The model under review builds one solid part; all positions refer to its coordinate system, in mm. Coordinates: 2 decimals unless noted, no trailing zeros. Loops run counter-clockwise (first coordinate to the right, second up) from the corner with the lowest first, then second, coordinate; pieces in that order, holes last. Notation, with made-up numbers: M 66,24 L 77,24 A13 ccw 77,28 Z; hole C 81.5,-20 d6. An arc over 180 degrees is marked long. Write item = value, one per line. Start each with the question number.
Q1. We need section A-A on x = 82.5. Give the boundary of the cut face in (y, z), and give its area (3 significant figures).
Q2. We need section B-B on z = 0.95. Count the separate pieces of the cut face and the enclosed holes in it, and give its area (3 significant figures).
Q3. Wall thickness on probe 1 along Y at (x, z) = (-24.5, 0.85); probe 2 along Y at (x, z) = (-123.5, 0.55) (3 decimals); probe 3 along Y at (x, z) = (-7.5, 0.65): over which ranges is each line inside the solid? List them lowest first.
Q4. Clearance check with a flat-ended pin moving along its axis: pin 1 Ø1 at (y, z) = (43, 1) entering from -X. State where the tip first meets the part, or that it passes through.
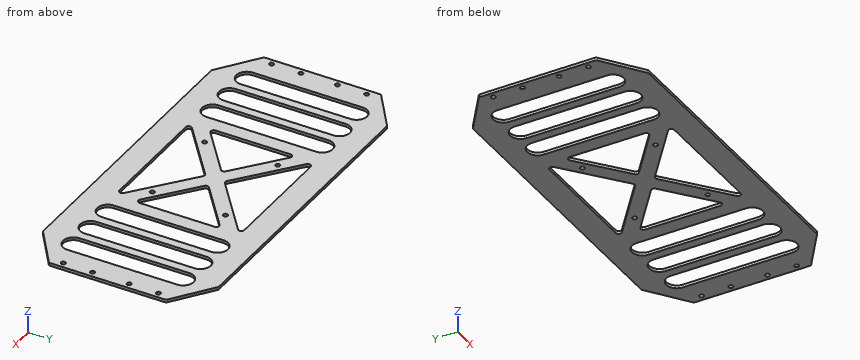
from build123d import *

# Parameters (mm, degrees)
EXTRUDE_1_DEPTH          = 2
SKETCH_2_R               = 1.525
CUT_EXTRUDE_1_DEPTH      = 1
CUT_EXTRUDE_1_DEPTH_BACK = 3
CUT_EXTRUDE_START        = -3
SKETCH_3_R               = 1.525
CUT_EXTRUDE_2_DEPTH      = 4
CUT_EXTRUDE_3_DEPTH      = 1
CUT_EXTRUDE_3_DEPTH_BACK = 3
FILLET_1_R               = 2
CUT_EXTRUDE_4_DEPTH      = 4
FILLET_2_R               = 2


with BuildPart() as part:
    # 草图1 → 凸台-拉伸1 (new body)
    with BuildSketch(Plane.XY):
        Polygon((-100, 60), (-127.5, 40), (-127.5, -40), (-100, -60), (100, -60), (127.5, -40), (127.5, 40), (100, 60), align=None)
    extrude(amount=EXTRUDE_1_DEPTH)

    # 草图2 → 切除-拉伸1 (cut, two sides)
    with BuildSketch(Plane(origin=(0, 0, 0), x_dir=(-1, 0, 0), z_dir=(0, 0, -1))) as cut_extrude_1_sk:
        with Locations((31, -25)):
            Circle(SKETCH_2_R)
        with Locations((-31, -25)):
            Circle(SKETCH_2_R)
        with Locations((-31, 25)):
            Circle(SKETCH_2_R)
        with Locations((31, 25)):
            Circle(SKETCH_2_R)
    extrude(amount=CUT_EXTRUDE_1_DEPTH, mode=Mode.SUBTRACT)
    extrude(cut_extrude_1_sk.sketch, amount=-CUT_EXTRUDE_1_DEPTH_BACK, mode=Mode.SUBTRACT)

    # 草图3 → 切除-拉伸2 (cut)
    with BuildSketch(Plane.XY.offset(2).offset(CUT_EXTRUDE_START)):
        with Locations((-123.5, -32.5)):
            Circle(SKETCH_3_R)
        with Locations((-123.5, -12.5)):
            Circle(SKETCH_3_R)
        with Locations((-123.5, 12.5)):
            Circle(SKETCH_3_R)
        with Locations((-123.5, 32.5)):
            Circle(SKETCH_3_R)
    cut_extrude_2 = extrude(amount=CUT_EXTRUDE_2_DEPTH, mode=Mode.SUBTRACT)

    # 镜向1: 切除-拉伸2 across plane
    add(cut_extrude_2.mirror(Plane(origin=(0, 0, 0), x_dir=(0, 0, 1), z_dir=(1, 0, 0))), mode=Mode.SUBTRACT)

    # 草图4 → 切除-拉伸3 (cut, two sides)
    with BuildSketch(Plane.XY.offset(2)) as cut_extrude_3_sk:
        Polygon((-45, 42.713647662), (45, 42.713647662), (0, 6.423325081), align=None)
        Polygon((-45, 29.866997499), (-45, -29.866997499), (-7.964923101, 0), align=None)
        Polygon((-45, -42.713647662), (45, -42.713647662), (0, -6.423325081), align=None)
        Polygon((45, -29.866997499), (7.964923101, 0), (45, 29.866997499), align=None)
    extrude(amount=CUT_EXTRUDE_3_DEPTH, mode=Mode.SUBTRACT)
    extrude(cut_extrude_3_sk.sketch, amount=-CUT_EXTRUDE_3_DEPTH_BACK, mode=Mode.SUBTRACT)

    # 圆角1
    fillet_1_edges = [part.edges().sort_by_distance(p)[0] for p in [
        (-45, 29.866997499, 1),
        (-7.964923101, 0, 1),
        (-45, -29.866997499, 1),
        (45, 29.866997499, 1),
        (45, -29.866997499, 1),
        (7.964923101, 0, 1),
        (0, 6.423325081, 1),
        (-45, 42.713647662, 1),
        (45, 42.713647662, 1),
        (-45, -42.713647662, 1),
        (0, -6.423325081, 1),
        (45, -42.713647662, 1),
    ]]
    fillet(fillet_1_edges, radius=FILLET_1_R)

    # 草图5 → 切除-拉伸4 (cut)
    with BuildSketch(Plane.XY.offset(2).offset(CUT_EXTRUDE_START)):
        with BuildLine():
            Line((-110, -37.5), (-110, 37.5))
            ThreePointArc((-110, 37.5), (-102.833333333, 44.666666667), (-95.666666667, 37.5))
            Line((-95.666666667, 37.5), (-95.666666667, -37.5))
            ThreePointArc((-95.666666667, -37.5), (-102.833333333, -44.666666667), (-110, -37.5))
        make_face()
        with BuildLine():
            Line((-75.333333333, 37.5), (-75.333333333, -37.5))
            ThreePointArc((-75.333333333, -37.5), (-82.5, -44.666666667), (-89.666666667, -37.5))
            Line((-89.666666667, -37.5), (-89.666666667, 37.5))
            ThreePointArc((-89.666666667, 37.5), (-82.5, 44.666666667), (-75.333333333, 37.5))
        make_face()
        with BuildLine():
            Line((-55, 37.5), (-55, -37.5))
            ThreePointArc((-55, -37.5), (-62.166666667, -44.666666667), (-69.333333333, -37.5))
            Line((-69.333333333, -37.5), (-69.333333333, 37.5))
            ThreePointArc((-69.333333333, 37.5), (-62.166666667, 44.666666667), (-55, 37.5))
        make_face()
    cut_extrude_4 = extrude(amount=CUT_EXTRUDE_4_DEPTH, mode=Mode.SUBTRACT)

    # 镜向2: 切除-拉伸4 across plane
    add(cut_extrude_4.mirror(Plane(origin=(0, 0, 0), x_dir=(0, 0, 1), z_dir=(1, 0, 0))), mode=Mode.SUBTRACT)

    # 圆角2
    fillet_2_edges = [part.edges().sort_by_distance(p)[0] for p in [
        (127.5, 40, 1),
        (127.5, -40, 1),
        (100, -60, 1),
        (-100, -60, 1),
        (-127.5, -40, 1),
        (-127.5, 40, 1),
        (-100, 60, 1),
        (100, 60, 1),
    ]]
    fillet(fillet_2_edges, radius=FILLET_2_R)


solid = part.part
Returned:
q1.outline = M -60,0 L -44.67,0 L -44.67,2 L -60,2 Z; M 44.67,0 L 60,0 L 60,2 L 44.67,2 Z
q1.area = 61.3 mm^2
q2.separate_pieces = 1
q2.enclosed_holes = 22
q2.area = 16,600 mm^2
q3.probe_1 = -60 to -42.71, -26.18 to -13.33, 13.33 to 26.18, 42.71 to 60
q3.probe_2 = -42.909 to -34.025, -30.975 to -14.025, -10.975 to 10.975, 14.025 to 30.975, 34.025 to 42.909
q3.probe_3 = -60 to -42.71, -12.47 to 12.47, 42.71 to 60
q4.pin_1 = -124.06
